Check sheet for the modelled part. Datum: model origin and axes. Units: mm. A direction names the side the tool comes from. Round coordinates to 2 decimals unless told otherwise and drop trailing zeros. Write each loop counter-clockwise with the first axis right and the second up, starting at its lowest first coordinate (ties: lowest second). Pieces come first, ordered by that corner, then holes.
Item 1: Release check for a two-part mould opening along X. For faces 6 (the flat face through (-1, 3, 0)), 7 (the cylindrical face through (-45.464, -1.479, -11.675)), 8 (the flat face through (-47, -1, 0)) record: +X half, -X half, draft (parallel to the pull), parting line (faces both ways), or undercut.
Item 2: Cross-section at C-C on x = 19.5. Enter the section's corners in (y, z), plus the area to 3 significant figures.
Item 3: Tool access check on faces 1 (the flat face through (-1, -1, -15)), 2 (the flat face through (42, 1, 0)), 3 (the flat face through (-42, 1, 0)), 4 (the flat face through (-1, 1, 10)), 5 (the flat face through (-1, 1, -10)). Record the directions out of +Z, -Z, +X, -X, +Y, -Y that give a thin tool (end or side, any length) a straight path to the whole face; none if there is none.
Item 4: Cross-section at D-D on z = 7.5. Enter the section's corners in (x, y), plus the area to 3 significant figures.
Item 5: Material ranges on line 1 (X direction, y = -1.35, z = -12); line 2 (X direction, y = 2.15, z = -0.25); line 3 (Z direction, x = -7, y = 2.05), recorded low to high.
Item 6: Cross-section at B-B on z = 12. Enter the section's corners in (x, y), plus the area to 3 significant figures.
Item 7: Go/stop test with flat-tipped pins: pin 1 Ø3.5 at (x, y) = (17, 2) entering from -Z; pin 2 Ø3.5 at (y, z) = (2, 3.5) entering from -X; pin 3 Ø0.9 at (y, z) = (2, 2.5) entering from +X. Record where each tip stops, or that it passes through.
Item 8: Cross-section at A-A on x = 44. Enter the section's corners in (y, z), plus the area to 3 significant figures.
from build123d import *

# Parameters (mm, degrees)
SKETCH1_W           = 84
SKETCH1_H           = 20
BOSS_EXTRUDE1_DEPTH = 3
SKETCH2_W           = 94
SKETCH2_H           = 30
SKETCH2_R           = 1.5
BOSS_EXTRUDE2_DEPTH = 3


with BuildPart() as part:
    # Sketch1 → Boss-Extrude1 (new body)
    with BuildSketch(Plane(origin=(0, 0, 0), x_dir=(1, 0, 0), z_dir=(0, 1, 0))):
        Rectangle(SKETCH1_W, SKETCH1_H)
    extrude(amount=BOSS_EXTRUDE1_DEPTH)

    # Sketch2 → Boss-Extrude2 (add)
    with BuildSketch(Plane.XZ):
        Rectangle(SKETCH2_W, SKETCH2_H)
        with Locations(Location((-44, 12, 0), (0, 0, 270))):
            Circle(SKETCH2_R, mode=Mode.SUBTRACT)
        with Locations(Location((-44, -12, 0), (0, 0, 270))):
            Circle(SKETCH2_R, mode=Mode.SUBTRACT)
        with Locations(Location((44, 12, 0), (0, 0, 270))):
            Circle(SKETCH2_R, mode=Mode.SUBTRACT)
        with Locations(Location((44, -12, 0), (0, 0, 270))):
            Circle(SKETCH2_R, mode=Mode.SUBTRACT)
    extrude(amount=BOSS_EXTRUDE2_DEPTH)


solid = part.part
Response values:
1. face 6: draft
1. face 7: undercut
1. face 8: -X half
2. outline: (-3, -15) - (0, -15) - (0, -10) - (3, -10) - (3, 10) - (0, 10) - (0, 15) - (-3, 15) - close
2. area: 150 mm2
3. face 1: -Z, +X, -X, +Y, -Y
3. face 2: +Z, -Z, +X, +Y
3. face 3: +Z, -Z, -X, +Y
3. face 4: +Z, +X, -X, +Y
3. face 5: -Z, +X, -X, +Y
4. outline: (-47, -3) - (47, -3) - (47, 0) - (42, 0) - (42, 3) - (-42, 3) - (-42, 0) - (-47, 0) - close
4. area: 534 mm2
5. line 1: x = -47 to -45.5, -42.5 to 42.5, 45.5 to 47
5. line 2: x = -42 to 42
5. line 3: z = -10 to 10
6. outline: (-47, -3) - (-45.5, -3) - (-45.5, 0) - (-47, 0) - close; (-42.5, -3) - (42.5, -3) - (42.5, 0) - (-42.5, 0) - close; (45.5, -3) - (47, -3) - (47, 0) - (45.5, 0) - close
6. area: 264 mm2
7. pin 1: stops at z = -10
7. pin 2: stops at x = -42
7. pin 3: stops at x = 42
8. outline: (-3, -15) - (0, -15) - (0, -13.5) - (-3, -13.5) - close; (-3, -10.5) - (0, -10.5) - (0, 10.5) - (-3, 10.5) - close; (-3, 13.5) - (0, 13.5) - (0, 15) - (-3, 15) - close
8. area: 72.0 mm2
